```python
from build123d import *

# Parameters (mm, degrees)
F1_DEPTH = 50.8


with BuildPart() as f1:
    # F0 (on Right) → F1 (new body)
    with BuildSketch(Plane.YZ):
        with BuildLine():
            Line((-8.452803, 0), (-2.102803, 0))
            Line((-2.102803, 0), (-2.102803, 1.5875))
            ThreePointArc((-2.102803, 1.5875), (1.072197, 4.7625), (4.247197, 1.5875))
            Line((4.247197, 1.5875), (4.247197, 0))
            Line((4.247197, 0), (10.597197, 0))
            Line((10.597197, 0), (10.597197, 0.79375))
            Line((10.597197, 0.79375), (5.040947, 0.79375))
            Line((5.040947, 0.79375), (5.040947, 1.5875))
            ThreePointArc((5.040947, 1.5875), (1.072197, 5.55625), (-2.896553, 1.5875))
            Line((-2.896553, 1.5875), (-2.896553, 0.79375))
            Line((-2.896553, 0.79375), (-8.452803, 0.79375))
            Line((-8.452803, 0.79375), (-8.452803, 0))
        make_face()
    extrude(amount=F1_DEPTH)


solid = f1.part
```
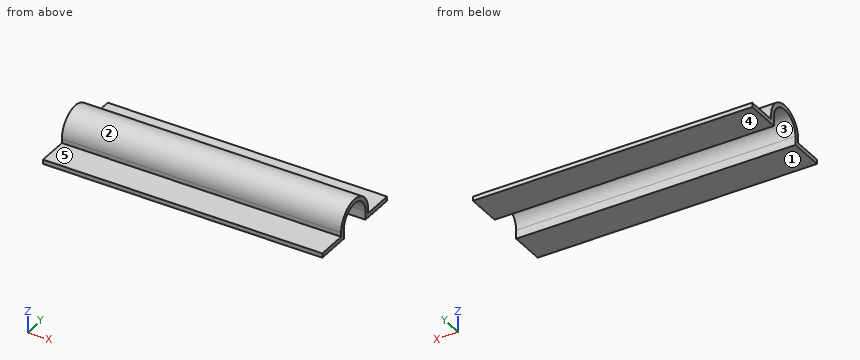
Geometry check sheet. Reference: the model listing, model coordinates, mm. Face numbers are marked on the shaded views. A direction names the side the tool comes from. Give positions to 0.01 mm unless a question says otherwise; leave off trailing zeros. Write each loop counter-clockwise with the first axis right and the second up, starting at its lowest first coordinate (ties: lowest second). Pieces come first, ordered by that corner, then holes. Notation, with made-up numbers: (-8, -8) -> (-1, -8) arc R36 cw to (-1, 27) -> close; hole circle Ø1 at (-28.5, 40.5). An arc over 180 degrees is marked (long way). Use one line per item in the form item = value.
Item 1: Access from +Z, -Z, +X, -X, +Y, -Y to the whole of each face (thin tool, end or side, straight path). Record for the marked faces 4 and 5.
Results list:
face_4 = -Z, +X, -X, +Y, -Y
face_5 = +Z, +X, -X, -Y
Item 2: Scan lines: line 1 (Y direction, x = 27.5, z = 0.75); line 2 (Y direction, x = 6.5, z = 1); line 3 (Z direction, x = 5.5, y = -7). Record each from-to range of solid material in increasing order.
Results list:
line_1 = -8.45 to -2.1, 4.25 to 10.6
line_2 = -2.9 to -2.1, 4.25 to 5.04
line_3 = 0 to 0.79
Item 3: Mould release check, pull along Y, two halves, no side actions. Record for the marked faces 1, 2 and 3: released by +Y, released by -Y, zero draft, split by the parting line, or undercut.
Results list:
face_1 = zero draft
face_2 = split by the parting line
face_3 = undercut
Item 4: Sectioned sample at D-D on y = 3.5. Enter the section's corners in (x, z), plus the area to 3 significant figures.
Results list:
outline = (0, 3.63) -> (50.8, 3.63) -> (50.8, 4.73) -> (0, 4.73) -> close
area = 55.5 mm2
Item 5: Sectioned sample at C-C on y = 7.5. Enter the section's corners in (x, z), plus the area to 3 significant figures.
Results list:
outline = (0, 0) -> (50.8, 0) -> (50.8, 0.79) -> (0, 0.79) -> close
area = 40.3 mm2
Item 6: Sectioned sample at B-B on z = 3.15. Enter the section's corners in (x, y).
Results list:
outline = (0, -2.58) -> (50.8, -2.58) -> (50.8, -1.69) -> (0, -1.69) -> close; (0, 3.84) -> (50.8, 3.84) -> (50.8, 4.72) -> (0, 4.72) -> close
Item 7: Depth check by flat-ended pin: pin 1 Ø3 at (x, z) = (23.5, 5) entering from -Y; pin 2 Ø3 at (x, y) = (17.5, -1.5) entering from +Z; pin 3 Ø3 at (x, y) = (27.5, -4.5) entering from +Z. Enter the tip coordinate at first touch or a pass-through.
Results list:
pin_1 = -2.41
pin_2 = 5.41
pin_3 = 0.79
